Work out the finished part from the listing and answer in its coordinate system (mm). Face numbers are marked on the shaded views. A direction names the side the tool comes from. Round coordinates to 2 decimals unless told otherwise and drop trailing zeros. Order: outer loops, then holes, each group sorted by start corner. A loop starts at its lowest first (then second) coordinate and runs counter-clockwise, first axis right, second up. Notation, with made-up numbers: (62.5, 2.5) -> (69.5, 2.5) arc R11 ccw to (69.5, 11.5) -> close; hole circle Ø2 at (14, 74.25). An arc over 180 degrees is marked (long way). Use a Markdown table: item, result. Add a question column.
Item 1: A tool of negligible diameter and unlimited length cuts with its end or side. For the marked faces 1 and 2, from which of +Z, -Z, +X, -X, +Y, -Y can it reach the whole face along a straight path? Write none if from no direction.
Item 2: Find the intervals of material crossed by L1, parallel to X at y = 59, z = 17; L2, parallel to Y at x = -26.5, z = -9.5; L3, parallel to Y at x = -45.5, z = 21, in increasing order. Write a range as [from, to].
Item 3: A cutting plane is placed at B-B, the plane y = 37.5. Determine the outline of the cut face in (x, z).
Item 4: A cutting plane is placed at C-C, the plane z = 35. Determine the outline of the cut face in (x, y).
Item 5: Flat-ended cylindrical pins translate along their axes: P1, Ø12, axis at x = -54.5, y = 44.5, coming from the -Z side; P2, Ø2.5, axis at x = -48.64, z = 49.04, coming from the -Y side; P3, Ø12, axis at x = 39, z = 56, coming from the +Y side. Find the tip coordinate at first contact, or state that the pin passes through.
Item 6: A cutting plane is placed at D-D, the plane y = 74.5. Determine the outline of the cut face in (x, z).
from build123d import *

# Parameters (mm, degrees)
SKETCH2_W           = 151
SKETCH2_H           = 152
BOSS_EXTRUDE1_DEPTH = 2
EXTRUDE_THIN1_DEPTH = 20
BOSS_EXTRUDE3_START = 75.5
BOSS_EXTRUDE3_DEPTH = 151
BOSS_EXTRUDE4_DEPTH = 2
BOSS_EXTRUDE5_DEPTH = 2
SKETCH8_R           = 25
CUT_EXTRUDE1_DEPTH  = 2
SKETCH9_W           = 80.4
SKETCH9_H           = 53
CUT_EXTRUDE6_DEPTH  = 10
SKETCH10_R          = 6.25
CUT_EXTRUDE7_DEPTH  = 10
SKETCH11_R          = 15
CUT_EXTRUDE8_DEPTH  = 10
SKETCH12_R          = 1.9
SKETCH12_R_2        = 1.27
CUT_EXTRUDE9_DEPTH  = 10
FILLET2_R           = 10
SKETCH15_W          = 18.5
SKETCH15_H          = 13
CUT_EXTRUDE12_DEPTH = 10
CUT_EXTRUDE13_DEPTH = 10
FILLET5_R           = 1
FILLET6_R           = 1
FILLET7_R           = 1
FILLET8_R           = 1
FILLET9_R           = 1
FILLET10_R          = 1
FILLET11_R          = 1
FILLET12_R          = 1
FILLET13_R          = 1
FILLET14_R          = 1
FILLET15_R          = 1
FILLET16_R          = 1
SKETCH19_R          = 1.5
CUT_EXTRUDE14_DEPTH = 10
FILLET17_R          = 10
FILLET19_R          = 10.42


with BuildPart() as part:
    # Sketch2 → Boss-Extrude1 (new body)
    with BuildSketch(Plane(origin=(0, 0, 0), x_dir=(1, 0, 0), z_dir=(0, 1, 0))):
        with Locations((0, -76)):
            Rectangle(SKETCH2_W, SKETCH2_H)
    extrude(amount=BOSS_EXTRUDE1_DEPTH)

    # Sketch3 → Extrude-Thin1 (add)
    with BuildSketch(Plane(origin=(0, 2, 0), x_dir=(1, 0, 0), z_dir=(0, 1, 0))):
        Polygon((-75.5, 0), (-75.5, -152), (75.5, -152), (75.5, 0), (73.5, 0), (73.5, -150), (-73.5, -150), (-73.5, 0), align=None)
    extrude(amount=EXTRUDE_THIN1_DEPTH)

    # Sketch4 → Boss-Extrude3 (add)
    with BuildSketch(Plane(origin=(0, 0, 0), x_dir=(0, 0, -1), z_dir=(1, 0, 0)).offset(BOSS_EXTRUDE3_START)):
        Polygon((0, 86), (23.969061552, 86), (23.969061552, 90), (0, 90), (-2.606060606, 90), (-152, 22), (-143.212121212, 22), (-2.606060606, 86), align=None)
    extrude(amount=-BOSS_EXTRUDE3_DEPTH)

    # Sketch6 → Boss-Extrude4 (add)
    with BuildSketch(Plane(origin=(75.5, 0, 0), x_dir=(0, 0, -1), z_dir=(1, 0, 0))):
        Polygon((0, 22), (-143.212121212, 22), (-2.606060606, 86), (0, 86), align=None)
    extrude(amount=-BOSS_EXTRUDE4_DEPTH)

    # Sketch7 → Boss-Extrude5 (add)
    with BuildSketch(Plane.ZY.offset(75.5)):
        Polygon((0, 86), (0, 22), (143.212121212, 22), (2.606060606, 86), align=None)
    extrude(amount=-BOSS_EXTRUDE5_DEPTH)

    # Sketch8 → Cut-Extrude1 (cut)
    with BuildSketch(Plane(origin=(75.5, 0, 0), x_dir=(0, 0, -1), z_dir=(1, 0, 0))):
        with Locations((-35, 35)):
            Circle(SKETCH8_R)
    extrude(amount=-CUT_EXTRUDE1_DEPTH, mode=Mode.SUBTRACT)

    # Sketch9 → Cut-Extrude6 (cut)
    with BuildSketch(Plane(origin=(0, 75.536424885, 34.382096844), x_dir=(1, 0, 0), z_dir=(0, 0.9101513920874156, 0.41427580605357506))):
        with Locations((-12.9, -45.503721555)):
            Rectangle(SKETCH9_W, SKETCH9_H)
    extrude(amount=-CUT_EXTRUDE6_DEPTH, mode=Mode.SUBTRACT)

    # Sketch10 → Cut-Extrude7 (cut)
    with BuildSketch(Plane(origin=(0, 75.536424885, 34.382096844), x_dir=(1, 0, 0), z_dir=(0, 0.9101513920874156, 0.41427580605357506))):
        with Locations(Location((55.95, -24.579806444, 0), (0, 0, 270))):
            Circle(SKETCH10_R)
    extrude(amount=-CUT_EXTRUDE7_DEPTH, mode=Mode.SUBTRACT)

    # Sketch11 → Cut-Extrude8 (cut)
    with BuildSketch(Plane(origin=(0, 75.536424885, 34.382096844), x_dir=(1, 0, 0), z_dir=(0, 0.9101513920874156, 0.41427580605357506))):
        with Locations(Location((57.5, -46.579806444, 0), (0, 0, 270))):
            Circle(SKETCH11_R)
    extrude(amount=-CUT_EXTRUDE8_DEPTH, mode=Mode.SUBTRACT)

    # Sketch12 → Cut-Extrude9 (cut)
    with BuildSketch(Plane(origin=(0, 75.536424885, 34.382096844), x_dir=(1, 0, 0), z_dir=(0, 0.9101513920874156, 0.41427580605357506))):
        with Locations(Location((67, -24.279806444, 0), (0, 0, 270))):
            Circle(SKETCH12_R)
        with Locations(Location((67, -75.079806444, 0), (0, 0, 270))):
            Circle(SKETCH12_R)
        with Locations(Location((-71.25, -24.279806444, 0), (0, 0, 270))):
            Circle(SKETCH12_R)
        with Locations(Location((-71.25, -75.079806444, 0), (0, 0, 270))):
            Circle(SKETCH12_R)
        with Locations(Location((55.5, -64.579806444, 0), (0, 0, 270))):
            Circle(SKETCH12_R_2)
    extrude(amount=-CUT_EXTRUDE9_DEPTH, mode=Mode.SUBTRACT)

    # Fillet2
    fillet2_edges = [part.edges().sort_by_distance(p)[0] for p in [
        (0, 22, 152),
    ]]
    fillet(fillet2_edges, radius=FILLET2_R)

    # Sketch15 → Cut-Extrude12 (cut)
    with BuildSketch(Plane.ZY.offset(75.5)):
        with Locations((29.25, 36.5)):
            Rectangle(SKETCH15_W, SKETCH15_H)
    extrude(amount=-CUT_EXTRUDE12_DEPTH, mode=Mode.SUBTRACT)

    # Sketch18 → Cut-Extrude13 (cut)
    with BuildSketch(Plane.ZY.offset(75.5)):
        Polygon((48.006551759, 19.1), (47.706551759, 19.1), (47.706551759, 5.6), (63.606551759, 5.6), (63.606551759, 19.1), align=None)
        Polygon((80.107551094, 20.95), (80.707551094, 20.95), (80.707551094, 6.575), (67.607551094, 6.534667741), (67.607551094, 20.95), align=None)
        Polygon((98.507551094, 20.95), (99.107551094, 20.95), (99.107551094, 6.575), (86.007551094, 6.575), (86.007551094, 20.95), align=None)
    extrude(amount=-CUT_EXTRUDE13_DEPTH, mode=Mode.SUBTRACT)

    # Fillet5
    fillet5_edges = [part.edges().sort_by_distance(p)[0] for p in [
        (-74.5, 20.95, 99.107551094),
    ]]
    fillet(fillet5_edges, radius=FILLET5_R)

    # Fillet6
    fillet6_edges = [part.edges().sort_by_distance(p)[0] for p in [
        (-74.5, 20.95, 86.007551094),
    ]]
    fillet(fillet6_edges, radius=FILLET6_R)

    # Fillet7
    fillet7_edges = [part.edges().sort_by_distance(p)[0] for p in [
        (-74.5, 6.575, 86.007551094),
    ]]
    fillet(fillet7_edges, radius=FILLET7_R)

    # Fillet8
    fillet8_edges = [part.edges().sort_by_distance(p)[0] for p in [
        (-74.5, 6.575, 99.107551094),
    ]]
    fillet(fillet8_edges, radius=FILLET8_R)

    # Fillet9
    fillet9_edges = [part.edges().sort_by_distance(p)[0] for p in [
        (-74.5, 20.95, 80.707551094),
    ]]
    fillet(fillet9_edges, radius=FILLET9_R)

    # Fillet10
    fillet10_edges = [part.edges().sort_by_distance(p)[0] for p in [
        (-74.5, 6.534667741, 67.607551094),
    ]]
    fillet(fillet10_edges, radius=FILLET10_R)

    # Fillet11
    fillet11_edges = [part.edges().sort_by_distance(p)[0] for p in [
        (-74.5, 20.95, 67.607551094),
    ]]
    fillet(fillet11_edges, radius=FILLET11_R)

    # Fillet12
    fillet12_edges = [part.edges().sort_by_distance(p)[0] for p in [
        (-74.5, 6.575, 80.707551094),
    ]]
    fillet(fillet12_edges, radius=FILLET12_R)

    # Fillet13
    fillet13_edges = [part.edges().sort_by_distance(p)[0] for p in [
        (-74.5, 19.1, 63.606551759),
    ]]
    fillet(fillet13_edges, radius=FILLET13_R)

    # Fillet14
    fillet14_edges = [part.edges().sort_by_distance(p)[0] for p in [
        (-74.5, 19.1, 47.706551759),
    ]]
    fillet(fillet14_edges, radius=FILLET14_R)

    # Fillet15
    fillet15_edges = [part.edges().sort_by_distance(p)[0] for p in [
        (-74.5, 5.6, 47.706551759),
    ]]
    fillet(fillet15_edges, radius=FILLET15_R)

    # Fillet16
    fillet16_edges = [part.edges().sort_by_distance(p)[0] for p in [
        (-74.5, 5.6, 63.606551759),
    ]]
    fillet(fillet16_edges, radius=FILLET16_R)

    # Sketch19 → Cut-Extrude14 (cut)
    with BuildSketch(Plane.XZ):
        with Locations(Location((9.358907141, 98.041860309, 0), (0, 0, 270))):
            Circle(SKETCH19_R)
        with Locations(Location((-48.641092859, 98.041860309, 0), (0, 0, 270))):
            Circle(SKETCH19_R)
        with Locations(Location((-48.641092859, 49.041860309, 0), (0, 0, 270))):
            Circle(SKETCH19_R)
        with Locations(Location((9.358907141, 49.041860309, 0), (0, 0, 270))):
            Circle(SKETCH19_R)
    extrude(amount=-CUT_EXTRUDE14_DEPTH, mode=Mode.SUBTRACT)

    # Fillet17
    fillet17_edges = [part.edges().sort_by_distance(p)[0] for p in [
        (0, 22, 143.212121212),
    ]]
    fillet(fillet17_edges, radius=FILLET17_R)

    # Fillet19
    # the kernel refuses this fillet: 10.42 mm, written as the material it adds along each edge
    with BuildSketch(Plane(origin=(-73.5, -24.05, 150), x_dir=(0, 0, -1), z_dir=(0, 1, 0))) as fillet19_piece_1_section:
        with BuildLine():
            CenterArc((FILLET19_R, -FILLET19_R), FILLET19_R, 90, 90)
            Line((0, -FILLET19_R), (0, 0))
            Line((0, 0), (FILLET19_R, 0))
        make_face()
    fillet19_piece_1 = extrude(amount=72.1, mode=Mode.PRIVATE)
    fillet19_piece_1 = split(fillet19_piece_1, bisect_by=Plane(origin=(-73.5, 11.537299555, 166.198357039), z_dir=(0, -0.9101513920874158, -0.41427580605357495)), keep=Keep.TOP, mode=Mode.PRIVATE)
    fillet19_piece_1 = split(fillet19_piece_1, bisect_by=Plane(origin=(-73.5, 0, 150), z_dir=(0, 1, 0)), keep=Keep.TOP, mode=Mode.PRIVATE)
    with BuildSketch(Plane(origin=(-73.5, -24.05, 150), x_dir=(0, 0, -1), z_dir=(0, 1, 0))) as fillet19_piece_2_section:
        with BuildLine():
            CenterArc((FILLET19_R, -FILLET19_R), FILLET19_R, 90, 90)
            Line((0, -FILLET19_R), (0, 0))
            Line((0, 0), (FILLET19_R, 0))
        make_face()
    fillet19_piece_2 = extrude(amount=72.1, mode=Mode.PRIVATE)
    fillet19_piece_2 = fillet19_piece_2 & Plane(origin=(-73.5, 15.564541031, 142), x_dir=(0, 0, 1), z_dir=(1, 0, 0)) * Cylinder(10, 186, mode=Mode.PRIVATE)
    with BuildSketch(Plane(origin=(73.5, -24.05, 150), x_dir=(-1, 0, 0), z_dir=(0, 1, 0))) as fillet19_piece_3_section:
        with BuildLine():
            CenterArc((FILLET19_R, -FILLET19_R), FILLET19_R, 90, 90)
            Line((0, -FILLET19_R), (0, 0))
            Line((0, 0), (FILLET19_R, 0))
        make_face()
    fillet19_piece_3 = extrude(amount=72.1, mode=Mode.PRIVATE)
    fillet19_piece_3 = split(fillet19_piece_3, bisect_by=Plane(origin=(73.5, 11.537299555, 166.198357039), z_dir=(0, -0.9101513920874158, -0.41427580605357495)), keep=Keep.TOP, mode=Mode.PRIVATE)
    fillet19_piece_3 = split(fillet19_piece_3, bisect_by=Plane(origin=(73.5, 0, 150), z_dir=(0, 1, 0)), keep=Keep.TOP, mode=Mode.PRIVATE)
    with BuildSketch(Plane(origin=(73.5, -24.05, 150), x_dir=(-1, 0, 0), z_dir=(0, 1, 0))) as fillet19_piece_4_section:
        with BuildLine():
            CenterArc((FILLET19_R, -FILLET19_R), FILLET19_R, 90, 90)
            Line((0, -FILLET19_R), (0, 0))
            Line((0, 0), (FILLET19_R, 0))
        make_face()
    fillet19_piece_4 = extrude(amount=72.1, mode=Mode.PRIVATE)
    fillet19_piece_4 = fillet19_piece_4 & Plane(origin=(73.5, 15.564541031, 142), x_dir=(0, 0, 1), z_dir=(1, 0, 0)) * Cylinder(10, 186, mode=Mode.PRIVATE)
    with BuildSketch(Plane(origin=(99.55, 2, 150), x_dir=(0, 1, 0), z_dir=(-1, 0, 0))) as fillet19_piece_5_section:
        with BuildLine():
            CenterArc((FILLET19_R, FILLET19_R), FILLET19_R, 180, 90)
            Line((0, FILLET19_R), (0, 0))
            Line((0, 0), (FILLET19_R, 0))
        make_face()
    fillet19_piece_5 = extrude(amount=199.1, mode=Mode.PRIVATE)
    fillet19_piece_5 = split(fillet19_piece_5, bisect_by=Plane(origin=(-75.5, 2, 150), z_dir=(1, 0, 0)), keep=Keep.TOP, mode=Mode.PRIVATE)
    fillet19_piece_5 = split(fillet19_piece_5, bisect_by=Plane(origin=(75.5, 2, 150), z_dir=(-1, 0, 0)), keep=Keep.TOP, mode=Mode.PRIVATE)
    with BuildSketch(Plane(origin=(97.446755584, 22, 150), x_dir=(0, 0.055144349629415036, -0.9984783927075983), z_dir=(-1, 0, 0))) as fillet19_piece_6_section:
        with BuildLine():
            CenterArc((9.875933547, 10.138731334), FILLET19_R, 183.161141999, 73.496080828)
            Line((-0.528211305, 9.564127211), (-1.56862579, 9.506666798))
            Line((-1.56862579, 9.506666798), (-1.040414485, -0.057460412))
            Line((-1.040414485, -0.057460412), (0.057460412, -1.040414485))
            ThreePointArc((0.057460412, -1.040414485), (4.669499422, -0.785699017), (7.230776161, -1.013873133))
            Line((7.230776161, -1.013873133), (7.471245014, 0))
        make_face()
    fillet19_piece_6 = extrude(amount=194.893511169, mode=Mode.PRIVATE)
    fillet19_piece_6 = split(fillet19_piece_6, bisect_by=Plane(origin=(-75.5, 22, 150), z_dir=(1, 0, 0)), keep=Keep.TOP, mode=Mode.PRIVATE)
    fillet19_piece_6 = split(fillet19_piece_6, bisect_by=Plane(origin=(75.5, 22, 150), z_dir=(-1, 0, 0)), keep=Keep.TOP, mode=Mode.PRIVATE)
    fillet19_piece_6 = fillet19_piece_6 & Plane(origin=(97.446755584, 15.564541031, 142), x_dir=(0, 0, 1), z_dir=(1, 0, 0)) * Cylinder(10, 429, mode=Mode.PRIVATE)
    add([fillet19_piece_1, fillet19_piece_2, fillet19_piece_3, fillet19_piece_4, fillet19_piece_5, fillet19_piece_6])


solid = part.part
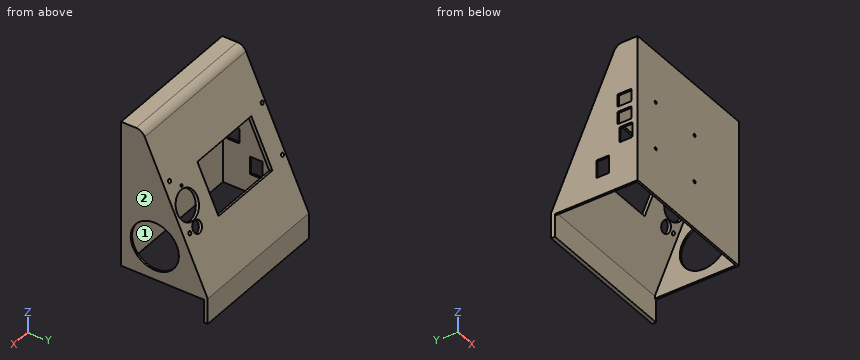
Reported:
| question | item | result |
|---|---|---|
| 1 | face 1 | -Z |
| 1 | face 2 | +Z, -Z, +X, +Y, -Y |
| 2 | L1 | [-75.5, -73.5], [73.5, 75.5] |
| 2 | L2 | [86, 90] |
| 2 | L3 | [0, 2], [77.63, 81.63] |
| 3 | outline | (-75.5, 0) -> (-73.5, 0) -> (-73.5, 20) -> (-75.5, 20) -> close; (-75.5, 38.5) -> (-73.5, 38.5) -> (-73.5, 109.16) -> (73.5, 109.16) -> (73.5, 59.87) -> (75.5, 59.87) -> (75.5, 117.95) -> (-75.5, 117.95) -> close; (73.5, 0) -> (75.5, 0) -> (75.5, 10.13) -> (73.5, 10.13) -> close |
| 4 | outline | (-75.5, 0) -> (75.5, 0) -> (75.5, 10) -> (73.5, 10) -> (73.5, 2) -> (-73.5, 2) -> (-73.5, 30) -> (-75.5, 30) -> close; (-75.5, 43) -> (-73.5, 43) -> (-73.5, 71.26) -> (73.5, 71.26) -> (73.5, 60) -> (75.5, 60) -> (75.5, 75.26) -> (-75.5, 75.26) -> close |
| 5 | P1 | z = 80.6 |
| 5 | P2 | y = 64.35 |
| 5 | P3 | y = 68.43 |
| 6 | outline | (-75.5, 0) -> (-73.5, 0) -> (-73.5, 27.87) -> (73.5, 27.87) -> (73.5, 0) -> (75.5, 0) -> (75.5, 36.66) -> (-75.5, 36.66) -> close |
